The model under review builds one solid part; all positions refer to its coordinate system, in mm. A direction names the side the tool comes from. Coordinates: 2 decimals unless noted, no trailing zeros. Loops run counter-clockwise (first coordinate to the right, second up) from the corner with the lowest first, then second, coordinate; pieces in that order, holes last. Notation, with made-up numbers: M 16.5,11.25 L 74.5,11.25 A37 ccw 74.5,50.25 Z; hole C 63.25,35.5 d9. An arc over 180 degrees is marked long. Use CSV: the item, a comma, the result in double quotes. Start each with the question number.
from build123d import *

# Parameters (mm, degrees)
F0_R          = 26.9875
F1_DEPTH      = 5.08
F0_R_2        = 23.8125
F0_W          = 165.1
F0_H          = 101.6
F3_DEPTH      = 76.2
F3_DEPTH_BACK = 76.2


with BuildPart() as f1:
    # F0 (on Top) → F1 (new body)
    with BuildSketch(Plane.XY):
        with BuildLine():
            Line((66.675, 36.5125), (-66.675, 36.5125))
            Line((-66.675, 36.5125), (-66.675, -9.55675))
            ThreePointArc((-66.675, -9.55675), (-58.779843617, -28.617343617), (-39.71925, -36.5125))
            Line((-39.71925, -36.5125), (39.6875, -36.5125))
            ThreePointArc((39.6875, -36.5125), (58.7705442573, -28.6080442573), (66.675, -9.525))
            Line((66.675, -9.525), (66.675, 36.5125))
        make_face()
        with Locations((-31.75, 0)):
            Circle(F0_R, mode=Mode.SUBTRACT)
        with Locations((31.75, 0)):
            Circle(F0_R, mode=Mode.SUBTRACT)
    extrude(amount=F1_DEPTH)



with BuildPart() as f1b:
    # F0 (on Top) → F1, piece 2 (new body)
    with BuildSketch(Plane.XY):
        with Locations((-31.75, 0)):
            Circle(F0_R_2)
    extrude(amount=F1_DEPTH)


with BuildPart() as f1c:
    # F0 (on Top) → F1, piece 3 (new body)
    with BuildSketch(Plane.XY):
        with Locations((31.75, 0)):
            Circle(F0_R_2)
    extrude(amount=F1_DEPTH)


with BuildPart() as f1d:
    # F0 (on Top) → F1, piece 4 (new body)
    with BuildSketch(Plane.XY):
        Rectangle(F0_W, F0_H)
        with BuildLine():
            Line((-73.025, -9.55675), (-73.025, 42.8625))
            Line((-73.025, 42.8625), (73.025, 42.8625))
            Line((73.025, 42.8625), (73.025, -9.525))
            ThreePointArc((73.025, -9.525), (63.2606723178, -33.0981723178), (39.6875, -42.8625))
            Line((39.6875, -42.8625), (-39.71925, -42.8625))
            ThreePointArc((-39.71925, -42.8625), (-63.2699716775, -33.1074716775), (-73.025, -9.55675))
        make_face(mode=Mode.SUBTRACT)
        with BuildLine():
            Line((73.025, 42.8625), (-73.025, 42.8625))
            Line((-73.025, 42.8625), (-73.025, -9.55675))
            ThreePointArc((-73.025, -9.55675), (-63.2699716775, -33.1074716775), (-39.71925, -42.8625))
            Line((-39.71925, -42.8625), (39.6875, -42.8625))
            ThreePointArc((39.6875, -42.8625), (63.2606723178, -33.0981723178), (73.025, -9.525))
            Line((73.025, -9.525), (73.025, 42.8625))
        make_face()
        with BuildLine():
            Line((-69.85, -9.55675), (-69.85, 39.6875))
            Line((-69.85, 39.6875), (69.85, 39.6875))
            Line((69.85, 39.6875), (69.85, -9.525))
            ThreePointArc((69.85, -9.525), (61.0156082875, -30.8531082875), (39.6875, -39.6875))
            Line((39.6875, -39.6875), (-39.71925, -39.6875))
            ThreePointArc((-39.71925, -39.6875), (-61.0249076472, -30.8624076472), (-69.85, -9.55675))
        make_face(mode=Mode.SUBTRACT)
    extrude(amount=F1_DEPTH)


with BuildPart() as f1_1:
    add(f1.part)

    add(f1b.part)  # F3 merges F1b

    add(f1c.part)  # F3 merges F1c

    add(f1d.part)  # F3 merges F1d
    # F2 (on Right) → F3 (join, two sides)
    with BuildSketch(Plane.YZ) as f3_sk:
        with BuildLine():
            Line((-0.9525, 0), (0.9525, 0))
            ThreePointArc((0.9525, 0), (0, 0.9525), (-0.9525, 0))
        make_face()
    extrude(amount=F3_DEPTH)
    extrude(f3_sk.sketch, amount=-F3_DEPTH_BACK)


solid = f1_1.part
1. Add section B-B (y = 7.5). Write out the cut boundary in (x, z) (3 decimals).
2. Add section A-A (z = 3.5). Give the number of separate pieces and of enclosed holes in the cut face, plus the area to 3 significant figures.
3. To check wall thickness, follow line 1 along Y through (x, z) = (31.75, 1.7); line 2 along Y through (x, z) = (-50.5, 2.75); line 3 along Y through (x, z) = (56, 3.6). State the ranges of each line that lie inside material, in increasing order.
4. Add section C-C (x = 31.75). Write out the cut boundary in (y, z), plus the area to 3 significant figures.
5. Add section D-D (y = -33). Write out the cut boundary in (x, z), plus the area to 3 significant figures.
6. Draft analysis for pull direction X (two halves, no side actions). For faces 1 (the flat face through (-82.55, -1, 3)), 2 (the cylindrical face through (-20.762, -21.126, 2.504)), 3 (the flat face through (-1, 1, 0)), state which applies: released by +X, released by -X, zero draft, split by the parting line, or undercut.
7. For faces 4 (the flat face through (-1, 39.688, 3)), 5 (the flat face through (-32, 0, 5.08)), list the 3-axis set-ups (+Z, -Z, +X, -X, +Y, -Y) from which the entire face can be reached by the end or side of a thin tool; tool diameter is ignored.
Solved:
1,outline,"M -82.55,0 L -69.85,0 L -69.85,5.08 L -82.55,5.08 Z; M -66.675,0 L -57.674,0 L -57.674,5.08 L -66.675,5.08 Z; M -54.351,0 L -9.149,0 L -9.149,5.08 L -54.351,5.08 Z; M -5.826,0 L 5.826,0 L 5.826,5.08 L -5.826,5.08 Z; M 9.149,0 L 54.351,0 L 54.351,5.08 L 9.149,5.08 Z; M 57.674,0 L 66.675,0 L 66.675,5.08 L 57.674,5.08 Z; M 69.85,0 L 82.55,0 L 82.55,5.08 L 69.85,5.08 Z"
2,separate pieces,"4"
2,enclosed holes,"3"
2,area,"14,500 mm^2"
3,line 1,"y = -50.8 to -39.69, -36.51 to -26.99, -23.81 to 23.81, 26.99 to 36.51, 39.69 to 50.8"
3,line 2,"y = -50.8 to -37.69, -34.26 to -19.41, -14.68 to 14.68, 19.41 to 36.51, 39.69 to 50.8"
3,line 3,"y = -50.8 to -34.9, -31.02 to -11.84, 11.84 to 36.51, 39.69 to 50.8"
4,outline,"M -50.8,0 L -39.69,0 L -39.69,5.08 L -50.8,5.08 Z; M -36.51,0 L -26.99,0 L -26.99,5.08 L -36.51,5.08 Z; M -23.81,0 L 23.81,0 L 23.81,5.08 L -23.81,5.08 Z; M 26.99,0 L 36.51,0 L 36.51,5.08 L 26.99,5.08 Z; M 39.69,0 L 50.8,0 L 50.8,5.08 L 39.69,5.08 Z"
4,area,"452 mm^2"
5,outline,"M -82.55,0 L -58.65,0 L -58.65,5.08 L -82.55,5.08 Z; M -53.02,0 L 53,0 L 53,5.08 L -53.02,5.08 Z; M 58.63,0 L 82.55,0 L 82.55,5.08 L 58.63,5.08 Z"
5,area,"782 mm^2"
6,face 1,"released by -X"
6,face 2,"undercut"
6,face 3,"zero draft"
7,face 4,"+Z, -Z"
7,face 5,"+Z, +X, -X, +Y, -Y"
